```python
from build123d import *

# Parameters (mm, degrees)
MODEL_W             = 77.14935
MODEL_H             = 96.19946
EXTRUDE_1_DEPTH     = 4
SKETCH_4_W          = 8
SKETCH_4_H          = 25
CUT_EXTRUDE_1_DEPTH = 227.33223095


with BuildPart() as part:
    # Model → 凸台-拉伸1 (new, symmetric)
    with BuildSketch(Plane.XY):
        Polygon((189.309527429, 123.984602236), (92.160177429, 123.984602236), (92.160177429, -5.214857764), (102.160177429, -5.214857764), (189.309527429, -5.214857764), align=None)
        with Locations((140.734852429, 45.884872236)):
            Rectangle(MODEL_W, MODEL_H, mode=Mode.SUBTRACT)
    extrude(amount=EXTRUDE_1_DEPTH, both=True)

    # 草图4 → 切除-拉伸1 (cut, through all)
    with BuildSketch(Plane.XY):
        with Locations((98.160177429, 29.884872236)):
            Rectangle(SKETCH_4_W, SKETCH_4_H)
        with Locations((183.309527429, 88.384872236)):
            Rectangle(SKETCH_4_W, SKETCH_4_H)
        with Locations((98.160177429, 88.384872236)):
            Rectangle(SKETCH_4_W, SKETCH_4_H)
        with Locations((183.309527429, 29.884872236)):
            Rectangle(SKETCH_4_W, SKETCH_4_H)
    extrude(amount=-CUT_EXTRUDE_1_DEPTH, mode=Mode.SUBTRACT)


solid = part.part
```
Could you check a few things on this model? Use its own coordinates, in mm. A direction names the side the tool comes from. Coordinates: 2 decimals unless noted, no trailing zeros. Write each loop counter-clockwise with the first axis right and the second up, starting at its lowest first coordinate (ties: lowest second). Pieces come first, ordered by that corner, then holes. Notation, with made-up numbers: M -37,6 L -22,6 A15 ccw -22,25 Z; hole C -18.75,8.25 d7. An arc over 180 degrees is marked long. Answer as CSV lines item,"result". Start each with the question number.
1) I want a section at D-D, the plane x = 100.5. Please give me the cut outline in (y, z), and give its area (3 significant figures).
2) I want a section at B-B, the plane x = 149.5. Please give me the cut outline in (y, z).
3) Please list where these lines run through material, in increasing order: line 1 (Y direction, x = 182, z = -1); line 2 (Y direction, x = 136, z = -0.5); line 3 (X direction, y = 21.5, z = 2.25). Write a range as from..to.
4) We'd pull the mould along Y, two halves only. Please class faces 1 (the flat face through (183, 17.385, -2)), 2 (the flat face through (140, 103, 4)): +Y half, -Y half, draft (parallel to the pull), parting line (faces both ways), or undercut.
5) For P1, Ø4, axis at x = 99.5, y = 25, coming from the -Z side; P2, Ø12, axis at x = 110.5, y = 48.5, coming from the -Z side, each with a flat end and sliding along its axis, tell me the tip position at first contact or that it passes through.
6) For faces 3 (the flat face through (92.16, 60, 0)), 4 (the flat face through (183, 100.885, -2)), 5 (the flat face through (140, 93.985, 0)), which set-ups out of +Z, -Z, +X, -X, +Y, -Y let a thin tool reach every point of the face, with its end or its side?
7) I want a section at A-A, the plane y = 67. Please give me the cut outline in (x, z).
8) I want a section at C-C, the plane z = 2.25. Please give me the cut outline in (x, y).
Data:
1,outline,"M -5.21,-4 L 17.38,-4 L 17.38,0 L 42.38,0 L 42.38,-4 L 75.88,-4 L 75.88,0 L 100.88,0 L 100.88,-4 L 123.98,-4 L 123.98,4 L -5.21,4 Z"
1,area,"834 mm^2"
2,outline,"M -5.21,-4 L -2.21,-4 L -2.21,4 L -5.21,4 Z; M 93.98,-4 L 123.98,-4 L 123.98,4 L 93.98,4 Z"
3,line 1,"y = -5.21..17.38, 42.38..75.88, 100.88..123.98"
3,line 2,"y = -5.21..-2.21, 93.98..123.98"
3,line 3,"x = 92.16..102.16, 179.31..189.31"
4,face 1,"undercut"
4,face 2,"draft"
5,P1,"stops at z = 0"
5,P2,"passes through"
6,face 3,"+Z, -Z, -X, +Y, -Y"
6,face 4,"-Z"
6,face 5,"+Z, -Z"
7,outline,"M 92.16,-4 L 102.16,-4 L 102.16,4 L 92.16,4 Z; M 179.31,-4 L 189.31,-4 L 189.31,4 L 179.31,4 Z"
8,outline,"M 92.16,-5.21 L 189.31,-5.21 L 189.31,123.98 L 92.16,123.98 Z; hole M 102.16,-2.21 L 179.31,-2.21 L 179.31,93.98 L 102.16,93.98 Z"
